The model under review builds one solid part; all positions refer to its coordinate system, in mm. A direction names the side the tool comes from. Round coordinates to 2 decimals unless told otherwise and drop trailing zeros. Write each loop counter-clockwise with the first axis right and the second up, starting at its lowest first coordinate (ties: lowest second). Pieces come first, ordered by that corner, then holes.
Item 1: Add section B-B (y = 18). Give the boundary of the cut face in (x, z) (3 decimals), plus the area to 3 significant figures.
Item 2: Add section D-D (x = 16.5). Give the boundary of the cut face in (y, z), plus the area to 3 significant figures.
Item 3: To check wall thickness, follow L1, parallel to Z at x = 0, y = 26; L2, parallel to Z at x = 0, y = 5.25 (3 decimals); L3, parallel to Z at x = -9, y = 2.5. State the ranges of each line that lie inside material, in increasing order.
Item 4: Machinability: for faces 1 (the face through (-7.4, 30, -3.6)), 2 (the face through (4.619, 6.902, -1.915)), 3 (the face through (7.678, 23.591, -2.418)), which of the approach directions +Z, -Z, +X, -X, +Y, -Y give a long, thin tool a straight path to every point of the face, cutting with its end or side? Answer none if there is none.
Item 5: Clearance check with flat-ended pins moving along their axes: pin 1 Ø6 at (x, z) = (4.5, 16.5) entering from -Y; pin 2 Ø4 at (y, z) = (14, 6.5) entering from -X; pin 3 Ø0.9 at (x, z) = (0.5, 14.5) entering from +Y; pin 4 Ø1.5 at (y, z) = (3, 4.5) entering from -X. State where each tip first meets the part, or that it passes through.
Item 6: Add section C-C (z = 7.5). Give the boundary of the cut face in (x, y).
Item 7: Add section A-A (z = 0). State how many separate pieces and enclosed holes the cut face has, plus the area to 3 significant figures.
Item 8: Draft analysis for pull direction X (two halves, no side actions). For faces 4 (the face through (-10, 10.1, -10)), 5 (the face through (-4, 0, -4)), 6 (the face through (-3.748, 25.07, 16.876)), 7 (the face through (3.3, 14, 0.1)), state which applies: +X half, -X half, draft (parallel to the pull), parting line (faces both ways), or undercut.
Autodesk Inventor part; units mm, degrees
ref_plane "Work Plane1" through (17.5, 0, 0) normal (1, 0, 0) x (0, 1, 0)
ref_plane "XZ Plane" through (0, 0, 0) normal (0, 1, 0) x (-1, 0, 0)
ref_plane "XY Plane" through (0, 0, 0) normal (0, 0, 1) x (1, 0, 0)
sketch "Sketch1" plane through (0, 0, 0) normal (0, 1, 0) x (-1, 0, 0)
  circle A0 centre (0, 0) radius 20.525
extrude "Extrusion1" add sketch "Sketch1" along normal blind 30
sketch "Sketch2" plane through (0, 30, 0) normal (0, 1, 0) x (1, 0, 0)
  circle A0 centre (0, 0) radius 8.05
  dimension "d3" = 16.1
extrude "Extrusion2" cut sketch "Sketch2" against normal blind 13
sketch "Sketch4" plane through (0, 17, 0) normal (0, 1, 0) x (1, 0, 0)
  circle A0 centre (0, 0) radius 3
  dimension "d27" = 6
sketch "Sketch5" plane through (0, 30, 0) normal (0, 1, 0) x (1, 0, 0)
  circle A0 centre (0, 0) radius 8.05
  circle A1 centre (0, 0) radius 20.525
  circle A2 centre (0, 14.2875) radius 1.5
extrude "Extrusion5" cut sketch "Sketch5" against normal blind 5 contours A2
pattern_circular "Circular Pattern2" count 4 over 360 about axis through (0, 0, 0) along (0, 1, 0) of "Extrusion5"
sketch "Sketch6" plane through (0, 30, 0) normal (0, 1, 0) x (1, 0, 0)
  circle A0 centre (0, 14.2875) radius 1.5
  line L0 (0, 15.7875) -> (0, 17.2875)
  circle A1 centre (0, 0) radius 17.2875
  circle A2 centre (0, 0) radius 20.525
  dimension "d22" = 1.5
extrude "Extrusion6" cut sketch "Sketch6" against normal blind 10 contours A2
extrude "Extrusion7" cut sketch "Sketch4" against normal blind 10
sketch "Sketch7" plane through (0, 0, 0) normal (0, -1, 0) x (1, 0, 0)
  circle A0 centre (0, 0) radius 5
  dimension "d28" = 10
extrude "Extrusion8" cut sketch "Sketch7" against normal blind 14
sketch "Sketch8" plane through (0, 30, 0) normal (0, 1, 0) x (1, 0, 0)
  circle A0 centre (0, 0) radius 17.2875
  circle A1 centre (14.2875, 0) radius 1.5
  circle A2 centre (0, -14.2875) radius 1.5
  circle A3 centre (-14.2875, 0) radius 1.5
  circle A4 centre (0, 14.2875) radius 1.5
  circle A5 centre (0, 0) radius 8.05
ref_plane "Work Plane1" through (17.5, 0, 0) normal (1, 0, 0) x (0, 1, 0)
sketch "Sketch9" plane through (17.5, 0, 0) normal (1, 0, 0) x (0, 1, 0)
  circle A0 centre (10, 0) radius 1.5
  dimension "d32" = 3
extrude "Extrusion9" cut sketch "Sketch9" along normal blind 50 and the other way blind 50
pattern_circular "Circular Pattern3" count 4 over 360 about axis through (0, 0, 0) along (0, 1, 0) of "Extrusion9"
sketch "Sketch10" plane through (0, 0, 0) normal (0, -1, 0) x (1, 0, 0)
  line L0 (-5.6922, -5.6922) -> (-7.7428, -3.6416)
  line L1 (-7.7428, -3.6416) -> (-18.2787, -14.1775)
  line L2 (-18.2787, -14.1775) -> (-14.1775, -18.2787)
  line L3 (-14.1775, -18.2787) -> (-3.6416, -7.7428)
  line L4 (-3.6416, -7.7428) -> (-5.6922, -5.6922)
  point P0 (0, 0)
extrude "Extrusion10" cut sketch "Sketch10" against normal blind 10.1
properties part number "tutup_syringe"
Numbers:
1. outline: circle Ø41.05 at (0, 0); hole circle Ø16.1 at (0, 0)
1. area: 1,120 mm2
2. outline: (0, -12.21) - (20, -12.21) - (20, -5.16) - (30, -5.16) - (30, 5.16) - (20, 5.16) - (20, 12.21) - (0, 12.21) - close; hole circle Ø3 at (10, 0)
2. area: 584 mm2
3. L1: z = -17.29 to -15.79, -12.79 to -8.05, 8.05 to 12.79, 15.79 to 17.29
3. L2: z = -20.525 to -5, 5 to 20.525
3. L3: z = -18.45 to -13.1, -4.9 to 18.45
4. face 1: +Z, -Z, +X, -X, +Y
4. face 2: -Y
4. face 3: +Y
5. pin 1: stops at y = 0
5. pin 2: stops at x = -20.03
5. pin 3: stops at y = 25
5. pin 4: stops at x = -20.18
6. outline: (-19.11, 0) - (19.11, 0) - (19.11, 20) - (15.58, 20) - (15.58, 30) - (2.92, 30) - (2.92, 17) - (-2.92, 17) - (-2.92, 30) - (-15.58, 30) - (-15.58, 20) - (-19.11, 20) - close; hole circle Ø3 at (0, 10)
7. separate pieces: 4
7. enclosed holes: 0
7. area: 676 mm2
8. face 4: undercut
8. face 5: draft
8. face 6: parting line
8. face 7: undercut
